Here's how the part is built. I have some questions about the finished solid (model axes, mm). Face numbers are marked on the shaded views. A direction names the side the tool comes from. Coordinates: 2 decimals unless noted, no trailing zeros. Write each loop counter-clockwise with the first axis right and the second up, starting at its lowest first coordinate (ties: lowest second). Pieces come first, ordered by that corner, then holes. Notation, with made-up numbers: (3, 76) -> (22, 76) arc R28 ccw to (22, 107) -> close; hole circle Ø4 at (57, 59.5). An arc over 180 degrees is marked (long way). Put each result on its own line as item: value. Start each with the question number.
Item 1: I need wall thicknesses on line 1 (X direction, y = 70, z = 12.75); line 2 (Y direction, x = -8.5, z = 13); line 3 (Y direction, x = -7, z = 7.25). Which ranges of each line are inside material? Lowest first, please. Write a range as [from, to].
Item 2: If we mould it in two halves opening along X, with no side actions, what happens to the marked faces 1, 2 and 3? For each: released by +X, released by -X, zero draft, split by the parting line, or undercut.
Item 3: I want a section at D-D, the plane z = 13.75. List the corners of the cut face in (x, y) for me, then the cut area to 4 significant figures.
Item 4: On a 3-axis mill with a long thin cutter (end or side, diameter ignored), from which of +Z, -Z, +X, -X, +Y, -Y can I reach the whole of each face in a straight line? I mean the marked faces 4, 5, 6 and 7. Say none if no direction works.
Item 5: For pin 1 (3 mm diameter, centred on x = -17, z = 5, fed in from +Y); pin 2 (2.5 mm diameter, centred on x = -16.5, y = 60, fed in from +Z); pin 3 (11 mm diameter, centred on x = -20, y = 24.5, fed in from -Z); pin 4 (11 mm diameter, centred on x = -16, y = 28, fed in from +Z), each with a flat end and sliding along its axis, tell me the tip position at first contact or that it passes through.
Item 6: I want a section at C-C, the plane y = 61. List the corners of the cut face in (x, z) for me, then the cut area to 3 significant figures.
Autodesk Inventor part; units mm, degrees
ref_plane "YZ Plane" through (0, 0, 0) normal (1, 0, 0) x (0, 1, 0)
ref_plane "XZ Plane" through (0, 0, 0) normal (0, 1, 0) x (-1, 0, 0)
ref_plane "XY Plane" through (0, 0, 0) normal (0, 0, 1) x (1, 0, 0)
sketch "Sketch1" plane through (0, 0, 0) normal (0, 0, 1) x (1, 0, 0)
  line L0 (0, 0) -> (-32, 0)
  line L1 (-32, 0) -> (-32, 76)
  line L2 (-32, 76) -> (0, 76)
  line L3 (0, 76) -> (0, 0)
  dimension "d0" = 32
  dimension "d1" = 76
extrude "Extrusion1" add sketch "Sketch1" along normal blind 16
fillet "Fillet1" radius 6 4 edges at (0, 76, 8) (-32, 76, 8) (0, 0, 8) (-32, 0, 8)
sketch "Sketch2" plane through (0, 0, 16) normal (0, 0, 1) x (1, 0, 0)
  line L0 (-6, 58) -> (-26, 58)
  line L1 (-26, 58) -> (-26, 18)
  line L2 (-26, 18) -> (-6, 18)
  line L3 (-6, 18) -> (-6, 58)
  line L4 (-6, 76) -> (-26, 76)
  line L5 (0, 6) -> (0, 70)
  point P0 (0, 0)
  dimension "d5" = 20
  dimension "d6" = 40
  dimension "d7" = 18
  dimension "d8" = 6
extrude "Extrusion2" cut sketch "Sketch2" against normal blind 10.5
sketch "Sketch3" plane through (0, 0, 5.5) normal (0, 0, 1) x (1, 0, 0)
  circle A0 centre (-16, 28) radius 7
  line L0 (-6, 58) -> (-6, 18)
  line L1 (-6, 18) -> (-26, 18)
  point P0 (0, 0)
  dimension "d11" = 14
  dimension "d12" = 10
  dimension "d13" = 10
extrude "Extrusion3" cut sketch "Sketch3" against normal up to surface (5.5 mm away)
sketch "Sketch4" plane through (0, 0, 16) normal (0, 0, 1) x (1, 0, 0)
  line L0 (-26, 58) -> (-6, 58)
  line L1 (-6, 58) -> (-26, 58)
  line L2 (-26, 58) -> (-26, 65.7)
  line L3 (-26, 65.7) -> (-6, 65.7)
  line L4 (-6, 65.7) -> (-6, 58)
  line L5 (-6, 18) -> (-26, 18)
  line L6 (-6, 18) -> (-26, 18)
  line L7 (-26, 18) -> (-26, 10.3)
  line L8 (-26, 10.3) -> (-6, 10.3)
  line L9 (-6, 10.3) -> (-6, 18)
  point P0 (0, 0)
  point P1 (-26, 18)
  dimension "d16" = 7.7
  dimension "d17" = 20
  dimension "d18" = 7.7
extrude "Extrusion4" cut sketch "Sketch4" against normal blind 5
sketch "Sketch5" plane through (0, 6, 0) normal (1, 0, 0) x (0, 0, -1)
  line L0 (0, -6) -> (-16, -6)
  line L1 (0, -6) -> (0, 4)
  line L2 (0, 0) -> (0, -6)
  line L3 (0, 4) -> (-10, 4)
  line L4 (-10, 4) -> (-10, -6)
  line L5 (0, 70) -> (0, 64)
  line L6 (0, 70) -> (-10, 70)
  line L7 (-10, 70) -> (-10, 60)
  line L8 (-10, 60) -> (0, 60)
  line L9 (0, 60) -> (0, 70)
  dimension "d21" = 10
  dimension "d22" = 10
  dimension "d23" = 10
  dimension "d24" = 10
extrude "Extrusion5" cut sketch "Sketch5" against normal up to surface (32 mm away)
fillet "Fillet2" radius 3 20 edges at (-16, 66, 0) (0, 38, 0) (-16, 10, 0) (-32, 38, 0) (0, 66, 5) (-32, 66, 5) (0, 10, 5) (-16, 66, 10) (-32, 10, 5) (-16, 10, 10) (-16, 76, 10) (-30.2426, 74.2426, 10) (-32, 68, 10) (0, 68, 10) (-1.7574, 74.2426, 10) (-1.7574, 1.7574, 10) (0, 8, 10) (-30.2426, 1.7574, 10) (-32, 8, 10) (-16, 0, 10)
sketch "Sketch6" plane through (-3, 69, 10) normal (0, 0, -1) x (-1, 0, 0)
  arc A0 (26, 1) -> (23, 4) centre (23, 1) ccw
  circle A1 centre (23, 1) radius 1.2
  arc A2 (3, 4) -> (0, 1) centre (3, 1) ccw
  circle A3 centre (3, 1) radius 1.2
  arc A4 (0, -63) -> (3, -66) centre (3, -63) ccw
  circle A5 centre (3, -63) radius 1.2
  arc A6 (23, -66) -> (26, -63) centre (23, -63) ccw
  circle A7 centre (23, -63) radius 1.2
  point P0 (-3, -69)
  dimension "d28" = 2.4
  dimension "d29" = 2.4
  dimension "d30" = 2.4
  dimension "d31" = 2.4
extrude "Extrusion6" cut sketch "Sketch6" along normal blind 5 and the other way blind 10
sketch "Sketch7" plane through (0, 0, 0) normal (0, 0, -1) x (-1, 0, 0)
  circle A0 centre (16, 28) radius 7
  circle A1 centre (16, 28) radius 11
  point P0 (0, 0)
  dimension "d36" = 22
extrude "Extrusion7" cut sketch "Sketch7" against normal blind 2
fillet "Fillet3" radius 2 1 edges at (-5, 28, 0)
properties part number "ramie03-7"
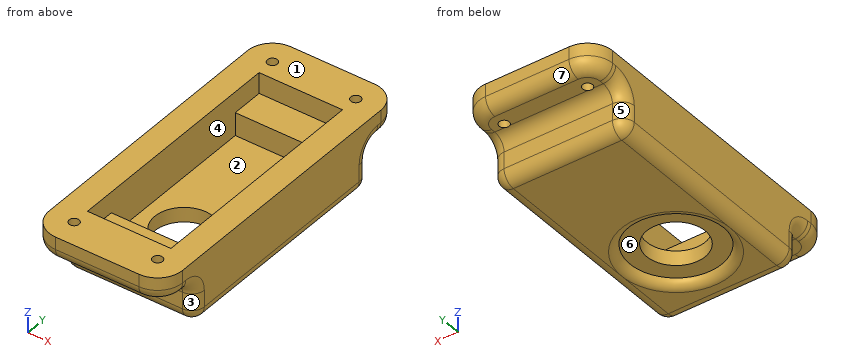
Calculated:
1. line 1: x = [-31.99, -27.2], [-24.8, -7.2], [-4.8, -0.01]
1. line 2: y = [0, 10.3], [65.7, 76]
1. line 3: y = [9.99, 18], [58, 66.01]
2. face 1: zero draft
2. face 2: undercut
2. face 3: released by +X
3. outline: (-32, 6) arc R6 ccw to (-26, 0) -> (-6, 0) arc R6 ccw to (0, 6) -> (0, 70) arc R6 ccw to (-6, 76) -> (-26, 76) arc R6 ccw to (-32, 70) -> close; hole circle Ø2.4 at (-26, 6); hole circle Ø2.4 at (-26, 70); hole (-26, 10.3) -> (-6, 10.3) -> (-6, 65.7) -> (-26, 65.7) -> close; hole circle Ø2.4 at (-6, 6); hole circle Ø2.4 at (-6, 70)
3. area: 1,275 mm2
4. face 4: +Z
4. face 5: -Z, -X, +Y
4. face 6: -Z
4. face 7: -Z, +X, -X, +Y
5. pin 1: stops at y = 66
5. pin 2: stops at z = 11
5. pin 3: stops at z = 2
5. pin 4: passes through
6. outline: (-32, 3) arc R3 ccw to (-29, 0) -> (-3, 0) arc R3 ccw to (0, 3) -> (0, 16) -> (-6, 16) -> (-6, 11) -> (-26, 11) -> (-26, 16) -> (-32, 16) -> close
6. area: 408 mm2
